Input: part model. Units: mm. Frame: model coordinates. A direction names the side the tool comes from. Coordinates: 2 decimals unless noted, no trailing zeros. Order: outer loops, then holes, each group sorted by start corner. A loop starts at its lowest first (then second) coordinate and runs counter-clockwise, first axis right, second up. Notation, with made-up numbers: M 87,39 L 122,39 A14 cw 122,48 Z; hole C 2.5,-39.5 d9. An arc over 180 degrees is marked long. Answer in a Markdown table with one row per item.
from build123d import *

# Parameters (mm, degrees)
SKETCH1_R           = 11.1010859
SKETCH1_RX          = 11.1010859
SKETCH1_RY          = 7.064327391
BOSS_EXTRUDE1_DEPTH = 3


with BuildPart() as part:
    # Sketch1 → Boss-Extrude1 (new body)
    with BuildSketch(Plane.XY):
        with BuildLine():
            Line((28.826197236, 15.137844409), (5.91044133, 15.137844409))
            ThreePointArc((5.91044133, 15.137844409), (3.673142738, 14.941061094), (1.504545567, 14.356753838))
            Line((1.504545567, 14.356753838), (-17.894214973, 7.255421854))
            ThreePointArc((-17.894214973, 7.255421854), (-21.907637047, 5.861214166), (-25.965065064, 4.60079768))
            ThreePointArc((-25.965065064, 4.60079768), (-29.412703897, 0), (-25.965065064, -4.60079768))
            ThreePointArc((-25.965065064, -4.60079768), (-21.907637047, -5.861214166), (-17.894214973, -7.255421854))
            Line((-17.894214973, -7.255421854), (1.504545567, -14.356753838))
            ThreePointArc((1.504545567, -14.356753838), (3.673142738, -14.941061094), (5.91044133, -15.137844409))
            Line((5.91044133, -15.137844409), (28.826197236, -15.137844409))
            Line((28.826197236, -15.137844409), (46.358712744, -15.137844409))
            ThreePointArc((46.358712744, -15.137844409), (46.397106085, -14.634708554), (46.434201657, -14.131475353))
            ThreePointArc((46.434201657, -14.131475353), (45.709460852, -13.733597625), (45.525288247, -12.927597395))
            ThreePointArc((45.525288247, -12.927597395), (45.896463104, -12.328004553), (46.569590651, -12.117810222))
            ThreePointArc((46.569590651, -12.117810222), (46.945219405, 0), (46.569590651, 12.117810222))
            ThreePointArc((46.569590651, 12.117810222), (45.752067528, 12.464773232), (45.525288247, 13.323434133))
            ThreePointArc((45.525288247, 13.323434133), (45.844356214, 13.879744795), (46.434201657, 14.131475353))
            ThreePointArc((46.434201657, 14.131475353), (46.397106085, 14.634708554), (46.358712744, 15.137844409))
            Line((46.358712744, 15.137844409), (28.826197236, 15.137844409))
        make_face()
        with Locations((-0.54553615, 0)):
            Circle(SKETCH1_R, mode=Mode.SUBTRACT)
        with Locations(Location((19.45446385, 0), (0, 0, -90))):
            Ellipse(SKETCH1_RX, SKETCH1_RY, mode=Mode.SUBTRACT)
        with BuildLine():
            Line((-16.54553615, -2.775271475), (-24.619053168, -2.775271475))
            ThreePointArc((-24.619053168, -2.775271475), (-27.394324643, 0), (-24.619053168, 2.775271475))
            Line((-24.619053168, 2.775271475), (-16.54553615, 2.775271475))
            ThreePointArc((-16.54553615, 2.775271475), (-13.770264675, 0), (-16.54553615, -2.775271475))
        make_face(mode=Mode.SUBTRACT)
    extrude(amount=BOSS_EXTRUDE1_DEPTH)


solid = part.part
1) Mould query, pull axis Y, two halves, no side actions, for faces 3 (the face through (-13.77, 0.06, 1.48)), 4 (the face through (25.2, 6.9, 3)), 5 (the face through (-8.059, 10.856, 1.479)). Classes: +Y half, -Y half, draft (parallel to the pull), parting line (faces both ways), or undercut.
Resolved:
| item | result |
|---|---|
| face 3 | undercut |
| face 4 | draft |
| face 5 | +Y half |
2) Reachability of faces 1 (the face through (25.2, 6.9, 0)), 2 (the face through (-21, -2.775, 1)) from +Z, -Z, +X, -X, +Y, -Y: full face, straight path, thin tool, end or side. Return the list, or none.
Resolved:
| item | result |
|---|---|
| face 1 | -Z, +X, -X, +Y, -Y |
| face 2 | +Z, -Z |
3) Material intervals for probe 1 along X at (y, z) = (3, 1.15); probe 2 along X at (y, z) = (2, 0.2) (3 decimals); probe 3 along Y at (x, z) = (18.5, 1.5), sorted ascending.
Resolved:
| item | result |
|---|---|
| probe 1 | x = -28.36 to -11.23, 10.14 to 12.65, 26.26 to 46.92 |
| probe 2 | x = -28.976 to -26.543, -14.621 to -11.465, 10.374 to 12.506, 26.403 to 46.935 |
| probe 3 | y = -15.14 to -11, 11 to 15.14 |
4) Cut plane A-A, the plane x = -7.5. Output: boundary loops of the cut face in (y, z).
Resolved:
| item | result |
|---|---|
| outline | M -11.06,0 L -8.65,0 L -8.65,3 L -11.06,3 Z; M 8.65,0 L 11.06,0 L 11.06,3 L 8.65,3 Z |
5) Cut plane B-B, the plane y = 0. State how many separate pieces and enclosed holes the cut face has, and give its area (3 significant figures).
Resolved:
| item | result |
|---|---|
| separate pieces | 4 |
| enclosed holes | 0 |
| area | 79.2 mm2 |
6) Contact query for flat-ended pins moving along their axis: pin 1 (5 mm diameter, centred on x = -11, y = -1.5, fed in from -Z); pin 2 (1 mm diameter, centred on x = -7.5, z = 2, fed in from -Y); pin 3 (1 mm diameter, centred on y = 4, z = 1.5, fed in from -X); pin 4 (2 mm diameter, centred on x = 15, y = -3.5, fed in from +Z). Output: stop coordinate, or through.
Resolved:
| item | result |
|---|---|
| pin 1 | stops at z = 0 |
| pin 2 | stops at y = -11.24 |
| pin 3 | stops at x = -27.89 |
| pin 4 | passes through |
